Read the model definition and answer for the solid it produces. Units are mm, in the model's axes. A direction names the side the tool comes from. Give positions to 0.01 mm unless a question says otherwise; leave off trailing zeros. Write each loop counter-clockwise with the first axis right and the second up, starting at its lowest first coordinate (ties: lowest second). Pieces come first, ordered by that corner, then holes. Notation, with made-up numbers: (83.5, 43.5) -> (97.5, 43.5) arc R14 ccw to (97.5, 59.5) -> close; hole circle Ø11 at (72, 7). An arc over 180 degrees is marked (long way). Use a Markdown table: item, result.
from build123d import *

# Parameters (mm, degrees)
BOSS_EXTRUDE1_DEPTH     = 13
CUT_EXTRUDE1_DEPTH      = 48.812132352
CUT_EXTRUDE2_DEPTH      = 48.812132352
CUT_EXTRUDE2_DEPTH_BACK = 48.812132352
SKETCH5_R               = 2.5
FILLET1_R               = 6.5
SKETCH6_R               = 2
CUT_EXTRUDE3_DEPTH      = 8


with BuildPart() as part:
    # Sketch2 → Boss-Extrude1 (new body)
    with BuildSketch(Plane.XY):
        Polygon((0, 0), (0, -34), (31, -34), (31, 0), (28, 0), (28, -15), (14, -15), (14, 0), align=None)
    extrude(amount=BOSS_EXTRUDE1_DEPTH)

    # Sketch4 → Cut-Extrude1 (cut, through all)
    with BuildSketch(Plane.ZY):
        with BuildLine():
            Line((4, -26.5), (4, -22.5))
            ThreePointArc((4, -22.5), (6.5, -20), (9, -22.5))
            Line((9, -22.5), (9, -26.5))
            ThreePointArc((9, -26.5), (6.5, -29), (4, -26.5))
        make_face()
    extrude(amount=-CUT_EXTRUDE1_DEPTH, mode=Mode.SUBTRACT)

    # Sketch5 → Cut-Extrude2 (cut, two sides: drawn at the far end of the back side and taken through both)
    with BuildSketch(Plane(origin=(31, 0, 0), x_dir=(0, 0, -1), z_dir=(1, 0, 0)).offset(-CUT_EXTRUDE2_DEPTH_BACK)):
        with Locations(Location((-6.5, -6.5, 0), (0, 0, 90))):
            Circle(SKETCH5_R)
    extrude(amount=CUT_EXTRUDE2_DEPTH + CUT_EXTRUDE2_DEPTH_BACK, mode=Mode.SUBTRACT)

    # Fillet1
    fillet1_edges = [part.edges().sort_by_distance(p)[0] for p in [
        (29.5, 0, 13),
        (7, 0, 13),
        (7, 0, 0),
        (29.5, 0, 0),
    ]]
    fillet(fillet1_edges, radius=FILLET1_R - 0.0001)  # a hair under: the kernel refuses the full size

    # Sketch6 → Cut-Extrude3 (cut)
    with BuildSketch(Plane.XZ.offset(34)):
        with Locations((15.5, 6.5)):
            Circle(SKETCH6_R)
    extrude(amount=-CUT_EXTRUDE3_DEPTH, mode=Mode.SUBTRACT)


solid = part.part
Item 1: A cutting plane is placed at D-D (y = -30). Give the vertices of the cut face in (x, z), then the cut area to 3 significant figures.
Return value:
| item | result |
|---|---|
| outline | (0, 0) -> (31, 0) -> (31, 13) -> (0, 13) -> close; hole circle Ø4 at (15.5, 6.5) |
| area | 390 mm^2 |
Item 2: A cutting plane is placed at B-B (z = 6). Give the vertices of the cut face in (x, y).
Return value:
| item | result |
|---|---|
| outline | (0, -34) -> (13.56, -34) -> (13.56, -28.95) -> (0, -28.95) -> close; (0, -20.05) -> (31, -20.05) -> (31, -8.95) -> (28, -8.95) -> (28, -15) -> (14, -15) -> (14, -8.95) -> (0, -8.95) -> close; (0, -4.05) -> (14, -4.05) -> (14, -0.02) -> (0, -0.02) -> close; (17.44, -34) -> (31, -34) -> (31, -28.95) -> (17.44, -28.95) -> close; (28, -4.05) -> (31, -4.05) -> (31, -0.02) -> (28, -0.02) -> close |
Item 3: A tool of negligible diameter and unlimited length cuts with its end or side. For faces 4 (the face through (15.3, -20, 6.4)), 5 (the face through (6.902, -1.854, 11.045)), 6 (the face through (21, -15, 6)), 7 (the face through (15, -34, 4)), 8 (the face through (17.408, -31.042, 7.101)), from which of +Z, -Z, +X, -X, +Y, -Y can it reach the whole face along a straight path? Write none if from no direction.
Return value:
| item | result |
|---|---|
| face 4 | +X, -X |
| face 5 | +Z, +X, -X, +Y |
| face 6 | +Z, -Z, +Y |
| face 7 | +Z, -Z, +X, -X, -Y |
| face 8 | -Y |
Item 4: Straight lines are drawn through the part: line 1 along Y through (x, z) = (28.85, 6.5); line 2 along X through (y, z) = (-12, 6.5); line 3 along X through (y, z) = (-29.75, 6.5). For each, find the intervals that lie inside material, in ascending order. Write a range as [from, to].
Return value:
| item | result |
|---|---|
| line 1 | [-34, -29], [-20, -9], [-4, 0] |
| line 2 | [0, 14], [28, 31] |
| line 3 | [0, 13.5], [17.5, 31] |
Item 5: For a pull along Y with two mould halves and no side action, classify faces 1 (the face through (29.479, -1.955, 11.146)), 2 (the face through (15, -25, 4)), 3 (the face through (15, -23, 13)) as +Y half, -Y half, draft (parallel to the pull), parting line (faces both ways), or undercut.
Return value:
| item | result |
|---|---|
| face 1 | +Y half |
| face 2 | undercut |
| face 3 | draft |
Item 6: This flat-tipped pin is pushed along its axis until it touches: P1, Ø4, axis at x = 23.5, z = 9, coming from the +Y side. Where does it stop, or does it pass through?
Return value:
| item | result |
|---|---|
| P1 | y = -15 |
Item 7: A cutting plane is placed at A-A (y = -11). Give the vertices of the cut face in (x, z), then the cut area to 3 significant figures.
Return value:
| item | result |
|---|---|
| outline | (0, 0) -> (14, 0) -> (14, 13) -> (0, 13) -> close; (28, 0) -> (31, 0) -> (31, 13) -> (28, 13) -> close |
| area | 221 mm^2 |
Item 8: A cutting plane is placed at C-C (x = 25). Give the vertices of the cut face in (y, z), then the cut area to 3 significant figures.
Return value:
| item | result |
|---|---|
| outline | (-34, 0) -> (-15, 0) -> (-15, 13) -> (-34, 13) -> close; hole (-26.5, 4) -> (-22.5, 4) arc R2.5 ccw to (-22.5, 9) -> (-26.5, 9) arc R2.5 ccw to start |
| area | 207 mm^2 |
